Input: part model. Units: mm. Frame: model coordinates. Face numbers are marked on the shaded views. A direction names the side the tool comes from. Round coordinates to 2 decimals unless told otherwise and drop trailing zeros. Loops run counter-clockwise (first coordinate to the right, second up) from the corner with the lowest first, then second, coordinate; pieces in that order, holes last. Notation, with made-up numbers: (45, 84) -> (98, 84) arc R14 cw to (98, 104) -> close; hole circle Ø9 at (28.25, 62). An arc over 180 degrees is marked (long way). Answer as a JSON object with one key per item and string values. Group by question number.
Item 1: Draft query along X for the marked faces 4, 5 and 6. Return one class per face: released by +X, released by -X, zero draft, split by the parting line, or undercut.
Item 2: Section query C-C on z = -11. Return loops of the section in (x, y), and give its area (3 significant figures).
Item 3: Section query D-D on x = -1. Return loops of the section in (y, z), and give its area (3 significant figures).
Item 4: Set-up query: the marked faces 1, 2 and 3. Return all of +Z, -Z, +X, -X, +Y, -Y with unobstructed straight access to the full face (end or side cutting, diameter ignored); none if empty.
Item 5: Section query A-A on x = -45.65. Return loops of the section in (y, z).
Item 6: Pin query (flat end, axial travel): pin 1 (8 mm diameter, centred on x = -9.5, z = -17, fed in from +Y); pin 2 (3 mm diameter, centred on x = -4, y = 7.5, fed in from -Z); pin 3 (4.5 mm diameter, centred on x = -62, y = 5, fed in from +Z); pin 4 (5 mm diameter, centred on y = 8.5, z = -4, fed in from +X). Return the tip coordinate at first contact, or that it passes through.
Item 7: Material intervals for line 1 (X direction, y = 6, z = -21.35) (3 decimals); line 2 (Z direction, x = -45.65, y = -2.5); line 3 (Z direction, x = -1, y = 9.25), sorted ascending. Write a range as [from, to].
Item 8: Section query B-B on y = 6. Count the separate pieces of the cut face and the enclosed holes in it, and give its area (3 significant figures).
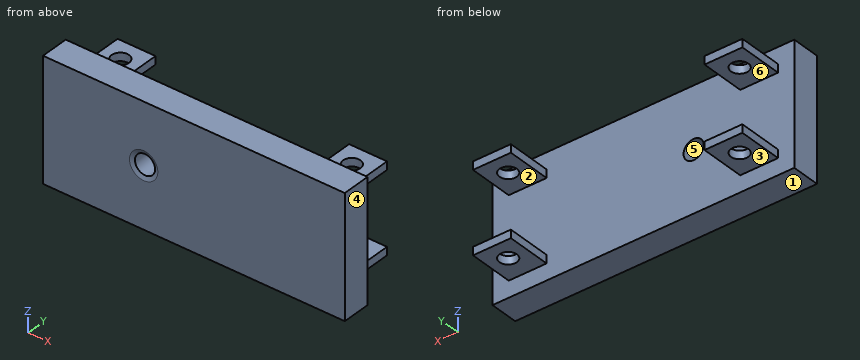
Autodesk Inventor part; units mm, degrees
ref_plane "YZ Plane" through (0, 0, 0) normal (1, 0, 0) x (0, 1, 0)
ref_plane "XZ Plane" through (0, 0, 0) normal (0, 1, 0) x (-1, 0, 0)
ref_plane "XY Plane" through (0, 0, 0) normal (0, 0, 1) x (1, 0, 0)
sketch "Sketch1" plane through (0, 0, 0) normal (0, 1, 0) x (-1, 0, 0)
  line L0 (0, 0) -> (66.5, 0)
  line L1 (66.5, 0) -> (66.5, -22)
  line L2 (66.5, -22) -> (0, -22)
  line L3 (0, -22) -> (0, 0)
  line L4 (66.5, -2) -> (0, -2)
  line L5 (66.5, -20) -> (0, -20)
  line L6 (9.35, 0) -> (9.35, -2)
  line L7 (9.35, -20) -> (9.35, -22)
  line L8 (59.65, 0) -> (59.65, -2)
  line L9 (59.65, -20) -> (59.65, -22)
  line L10 (57.15, -22) -> (57.15, -20)
  line L11 (64, -22) -> (64, -20)
  line L12 (2.5, -22) -> (2.5, -20)
  line L13 (6.85, -22) -> (6.85, -20)
  line L14 (0, -11) -> (66.5, -11)
  line L15 (9.35, -2) -> (9.35, 0)
  line L16 (59.65, -2) -> (59.65, 0)
  line L17 (57.15, 0) -> (57.15, -2)
  line L18 (64, 0) -> (64, -2)
  line L19 (2.5, 0) -> (2.5, -2)
  line L20 (6.85, 0) -> (6.85, -2)
  line L21 (33.25, -2) -> (33.25, -20)
  line L22 (66.5, -22) -> (0, -22)
  line L23 (0, -22) -> (0, -26)
  line L24 (0, -26) -> (66.5, -26)
  line L25 (66.5, -26) -> (66.5, -22)
  line L26 (66.5, 0) -> (0, 0)
  line L27 (0, 0) -> (0, 4)
  line L28 (0, 4) -> (66.5, 4)
  line L29 (66.5, 4) -> (66.5, 0)
  line L30 (66.5, -26) -> (70.5, -26)
  line L31 (70.5, -26) -> (70.5, 4)
  line L32 (70.5, 4) -> (66.5, 4)
  line L33 (66.5, 4) -> (66.5, -26)
  line L34 (0, -26) -> (-4, -26)
  line L35 (-4, -26) -> (-4, 4)
  line L36 (-4, 4) -> (0, 4)
  line L37 (0, 4) -> (0, -26)
  point P0 (2.5, -21)
  point P1 (57.15, -21)
  point P2 (59.65, -21)
  point P3 (64, -21)
  point P4 (6.85, -21)
  point P5 (57.15, -2)
  point P6 (33.25, -11)
  point P7 (0, -22)
  point P8 (0, -22)
  dimension "d2" = 2
  dimension "d3" = 2
  dimension "d36" = 18
  dimension "d38" = 4.35
  dimension "d39" = 4.35
  dimension "d40" = 61.5
  dimension "d41" = 2.5
  dimension "d42" = 2.5
  dimension "d43" = 2.5
  dimension "d44" = 2.5
  dimension "d67" = 4
  dimension "d68" = 4
  dimension "d71" = 4
  dimension "d72" = 4
extrude "Extrusion2" add sketch "Sketch1" against normal blind 7 contours L0 L19 L4 L3 | L0 L20 L4 L19 | L4 L21 L14 L3 | L0 L6 L4 L20 | L14 L21 L5 L3 | L0 L17 L4 L6 | L5 L12 L2 L3 | L21 L4 L1 L14 | L14 L1 L5 L21 | L1 L4 L18 L0 | L0 L8 L4 L17 | L5 L13 L2 L12 | L5 L10 L2 L7 | L18 L4 L8 L0 | L5 L7 L2 L13 | L1 L2 L11 L5 | L5 L9 L2 L10 | L11 L2 L9 L5
extrude "Extrusion5" add sketch "Sketch1" along normal blind 11 contours L0 L19 L4 L3 | L0 L20 L4 L19 | L0 L6 L4 L20 | L5 L12 L2 L3 | L1 L4 L18 L0 | L0 L8 L4 L17 | L5 L13 L2 L12 | L18 L4 L8 L0 | L5 L7 L2 L13 | L1 L2 L11 L5 | L5 L9 L2 L10 | L11 L2 L9 L5
sketch "Sketch5" plane through (-66.5, -7, 0) normal (0, 0, 1) x (1, 0, 0)
  point P0 (66.5, 7)
sketch "Sketch6" plane through (-66.5, -7, 0) normal (0, 0, 1) x (1, 0, 0)
  point P0 (66.5, 7)
sketch "Sketch7" plane through (-66.5, -7, 0) normal (0, 0, 1) x (1, 0, 0)
  line L0 (66.5, 0) -> (66.5, 18)
  line L1 (57.15, 18) -> (66.5, 18)
  line L2 (0, 18) -> (9.35, 18)
  line L3 (9.35, 7) -> (9.35, 18)
  point P0 (66.5, 7)
  point P1 (61.825, 13)
  point P2 (4.675, 13)
  dimension "d55" = 4.675
  dimension "d56" = 5
  dimension "d57" = 5
  dimension "d58" = 4.675
sketch "Sketch8" plane through (0, -7, -22) normal (0, 0, -1) x (-1, 0, 0)
  point P0 (0, 7)
  point P1 (4.675, 13)
  point P2 (61.825, 13)
hole "Hole3" at (-4.675, 6, -22) at (-61.825, 6, -22) direction (0, 0, 1) diameter 4.3 end through all
extrude "Extrusion6" add sketch "Sketch1" against normal blind 7 contours L27 L28 L29 L0 | L2 L25 L24 L23
extrude "Extrusion7" add sketch "Sketch1" against normal blind 7 contours L3 L23 L34 L35 L36 L27 | L32 L31 L30 L25 L1 L29
sketch "Sketch9" plane through (0, -7, 0) normal (0, -1, 0) x (1, 0, 0)
  line L0 (-70.5, 4) -> (4, 4)
  line L1 (4, -26) -> (-70.5, -26)
  line L2 (-70.5, -26) -> (-70.5, 4)
  line L3 (4, -26) -> (4, 4)
  line L4 (4, 4) -> (-70.5, 4)
  line L5 (-45.65, 4) -> (-45.65, -26)
  line L6 (-70.5, -11) -> (4, -11)
  line L7 (4, 4) -> (4, -26)
  point P0 (0, 0)
  point P1 (-33.25, -11)
  point P2 (-45.65, -11)
  dimension "d91" = 24.85
hole "Hole4" at (-45.65, -7, -11) direction (0, 1, 0) diameter 4.9784 end through all countersink diameter 7 countersink angle 135
properties part number "RadarMount_3DPrint"
Solved:
{
 "1": {"face 4": "released by +X", "face 5": "undercut", "face 6": "zero draft"},
 "2": {"outline": "(-70.5, -7) -> (-49.15, -7) -> (-48.14, -6.58) -> (-48.14, 0) -> (-70.5, 0) -> close; (-43.16, -6.58) -> (-42.15, -7) -> (4, -7) -> (4, 0) -> (-43.16, 0) -> close", "area": "486 mm²"},
 "3": {"outline": "(-7, -26) -> (0, -26) -> (0, -22) -> (11, -22) -> (11, -20) -> (0, -20) -> (0, -2) -> (11, -2) -> (11, 0) -> (0, 0) -> (0, 4) -> (-7, 4) -> close", "area": "254 mm²"},
 "4": {"face 1": "-Z, +X, -X, +Y, -Y", "face 2": "+X, -X, +Y", "face 3": "-Z, +X, -X, +Y"},
 "5": {"outline": "(-7, -26) -> (0, -26) -> (0, -13.49) -> (-6.58, -13.49) -> (-7, -14.5) -> close; (-7, -7.5) -> (-6.58, -8.51) -> (0, -8.51) -> (0, 4) -> (-7, 4) -> close"},
 "6": {"pin 1": "y = 11", "pin 2": "z = -22", "pin 3": "z = 0", "pin 4": "x = 0"},
 "7": {"line 1": "[-66.5, -63.975], [-59.675, -57.15], [-9.35, -6.825], [-2.525, 0]", "line 2": "[-26, -13.49], [-8.51, 4]", "line 3": "[-22, -20], [-2, 0]"},
 "8": {"separate pieces": "8", "enclosed holes": "0", "area": "40.4 mm²"}
}
